Geometry: see drawing. Coordinates: mm, zero at the bounding-box minimum. A direction names the side the tool comes from. Round coordinates to 2 decimals unless told otherwise and drop trailing zeros. Order: outer loops, then holes, each group sorted by start corner. A loop starts at its lowest first (then second) coordinate and runs counter-clockwise, first axis right, second up. Notation, with made-up numbers: (52.25, 27) -> (69.25, 27) arc R16 ccw to (69.25, 46) -> close; hole circle Ø3 at (1, 50). An arc over 180 degrees is marked (long way). Put each result on its own line as item: value.
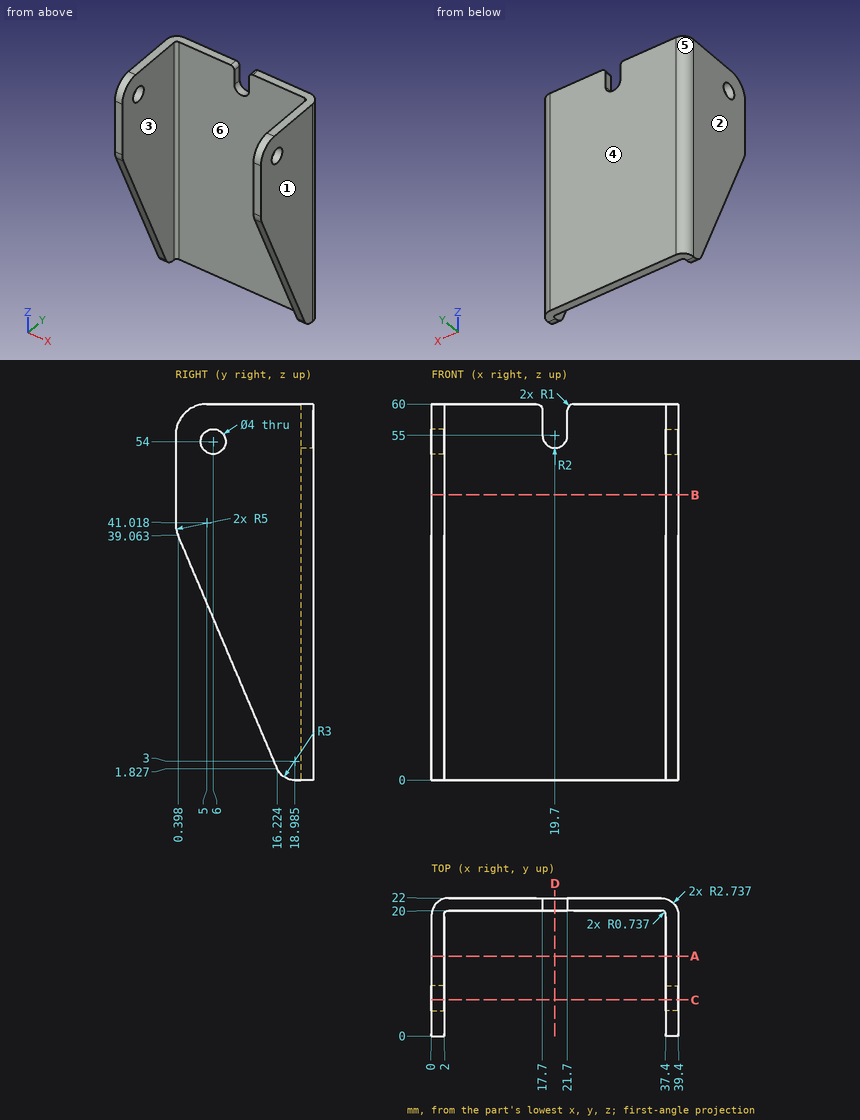
1. Cut plane C-C on y = 5.75. Return loops of the section in (x, z) (1 decimal), and give its area (3 significant figures).
Ans:
outline: (0, 26.5) -> (2, 26.5) -> (2, 52) -> (0, 52) -> close; (0, 56) -> (2, 56) -> (2, 60) -> (0, 60) -> close; (37.4, 26.5) -> (39.4, 26.5) -> (39.4, 52) -> (37.4, 52) -> close; (37.4, 56) -> (39.4, 56) -> (39.4, 60) -> (37.4, 60) -> close
area: 118 mm²
2. Draft query along X for the marked faces 1, 2, 3 and 4. Return one class per face: +X half, -X half, draft (parallel to the pull), parting line (faces both ways), or undercut.
Ans:
face 1: +X half
face 2: -X half
face 3: undercut
face 4: draft
3. Contact query for flat-ended pins moving along their axis: P1, Ø10, axis at x = 11.5, z = 30, coming from the -Y side; P2, Ø0.6, axis at y = 21, z = 56.5, coming from the +X side; P3, Ø1.6, axis at y = 20.5, z = 56.5, coming from the -X side (1 decimal); P4, Ø2.5, axis at y = 6, z = 54, coming from the -X side. Output: stop coordinate, or through.
Ans:
P1: y = 20
P2: x = 38.99
P3: x = 0
P4: through
4. Set-up query: the marked faces 5 and 6. Return all of +Z, -Z, +X, -X, +Y, -Y with unobstructed straight access to the full face (end or side cutting, diameter ignored); none if empty.
Ans:
face 5: +Z, -Z, -X, +Y
face 6: +Z, -Z, -Y
5. Cut plane B-B on z = 45.5. Return loops of the section in (x, y), and give its area (3 significant figures).
Ans:
outline: (0, 0) -> (2, 0) -> (2, 19.26) arc R0.74 cw to (2.74, 20) -> (36.66, 20) arc R0.74 cw to (37.4, 19.26) -> (37.4, 0) -> (39.4, 0) -> (39.4, 19.26) arc R2.74 ccw to (36.66, 22) -> (2.74, 22) arc R2.74 ccw to (0, 19.26) -> close
area: 156 mm²
6. Material intervals for probe 1 along X at (y, z) = (10.5, 48); probe 2 along Y at (x, z) = (9.5, 20.5); probe 3 along Z at (x, y) = (0.7, 6) (1 decimal), sorted ascending.
Ans:
probe 1: 0 to 2, 37.4 to 39.4
probe 2: 20 to 22
probe 3: 25.9 to 52, 56 to 60
7. Cut plane D-D on x = 19.7. Return loops of the section in (y, z).
Ans:
outline: (20, 0) -> (22, 0) -> (22, 53) -> (20, 53) -> close
8. Cut plane A-A on y = 12.75. Return loops of the section in (x, z), and give its area (3 significant figures).
Ans:
outline: (0, 10) -> (2, 10) -> (2, 60) -> (0, 60) -> close; (37.4, 10) -> (39.4, 10) -> (39.4, 60) -> (37.4, 60) -> close
area: 200 mm²
